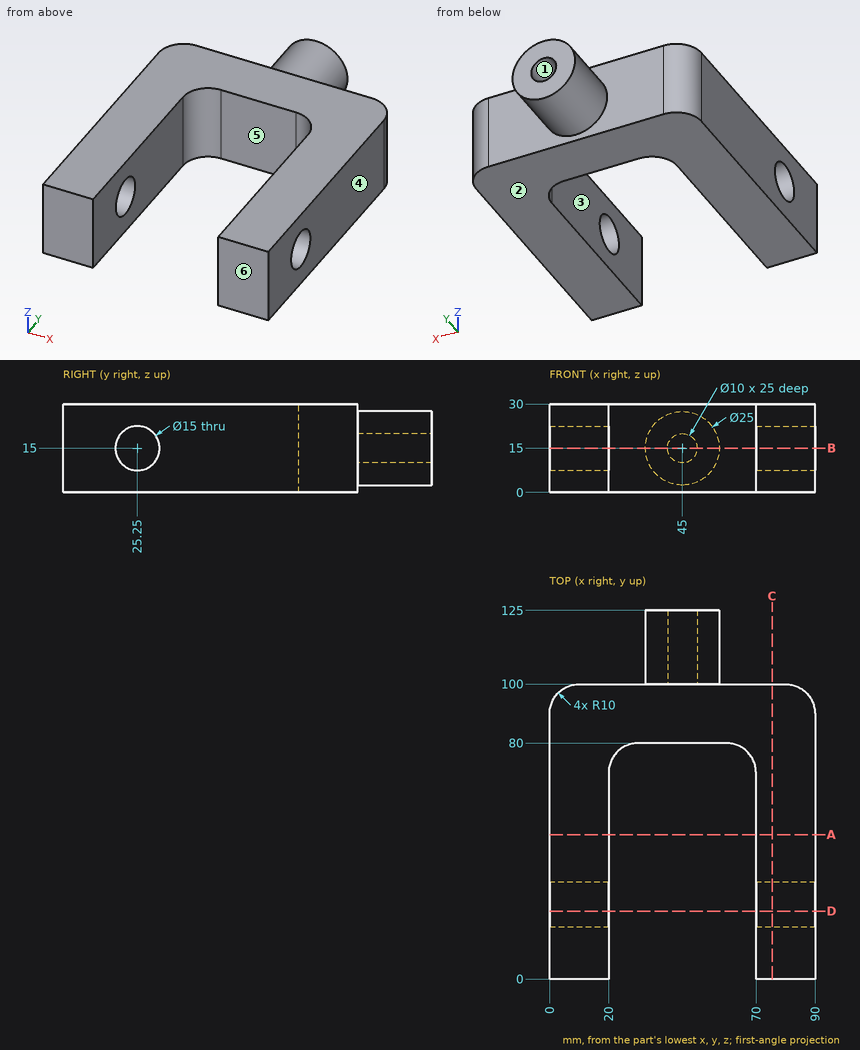
Source: three-view drawing plus pictorial views. Frame: mm from the lowest corner of the part. A direction names the side the tool comes from. Round coordinates to 2 decimals unless told otherwise and drop trailing zeros. Order: outer loops, then holes, each group sorted by start corner. A loop starts at its lowest first (then second) coordinate and runs counter-clockwise, first axis right, second up. Notation, with made-up numbers: (11, 16) - (15, 16) arc R18 ccw to (15, 26) - close; hole circle Ø4 at (-7.5, 58). An arc over 180 degrees is marked (long way). Write each question's results on one line, items separated by ' | '.
Item 1: Material intervals for line 1 along X through (y, z) = (11.5, 15.5); line 2 along X through (y, z) = (116, 15); line 3 along Y through (x, z) = (79.5, 27.75), sorted ascending. Write a range as [from, to].
Completed:
line 1: [0, 20], [70, 90] | line 2: [32.5, 40], [50, 57.5] | line 3: [0, 100]
Item 2: Section D-D, the plane y = 23. Return the cut outline in (x, z), and give its area (3 significant figures).
Completed:
outline: (0, 0) - (20, 0) - (20, 7.85) - (0, 7.85) - close; (0, 22.15) - (20, 22.15) - (20, 30) - (0, 30) - close; (70, 0) - (90, 0) - (90, 7.85) - (70, 7.85) - close; (70, 22.15) - (90, 22.15) - (90, 30) - (70, 30) - close | area: 628 mm^2
Item 3: Section A-A, the plane y = 49. Return the cut outline in (x, z), and give its area (3 significant figures).
Completed:
outline: (0, 0) - (20, 0) - (20, 30) - (0, 30) - close; (70, 0) - (90, 0) - (90, 30) - (70, 30) - close | area: 1,200 mm^2
Item 4: Section B-B, the plane z = 15. Return the cut outline in (x, y).
Completed:
outline: (0, 0) - (20, 0) - (20, 17.75) - (0, 17.75) - close; (0, 32.75) - (20, 32.75) - (20, 70) arc R10 cw to (30, 80) - (60, 80) arc R10 cw to (70, 70) - (70, 32.75) - (90, 32.75) - (90, 90) arc R10 ccw to (80, 100) - (57.5, 100) - (57.5, 125) - (50, 125) - (50, 100) - (40, 100) - (40, 125) - (32.5, 125) - (32.5, 100) - (10, 100) arc R10 ccw to (0, 90) - close; (70, 0) - (90, 0) - (90, 17.75) - (70, 17.75) - close
Item 5: Section C-C, the plane x = 75.5. Return the cut outline in (y, z), and give its area (3 significant figures).
Completed:
outline: (0, 0) - (100, 0) - (100, 30) - (0, 30) - close; hole circle Ø15 at (25.25, 15) | area: 2,820 mm^2
Item 6: Mould query, pull axis X, two halves, no side actions, for the marked faces 4, 5 and 6. Classes: pulls with the +X half, pulls with the -X half, needs draft (parallel to the pull), parting line crosses it, or undercut.
Completed:
face 4: pulls with the +X half | face 5: undercut | face 6: needs draft
Item 7: Reachability of the marked faces 1, 2 and 3 from +Z, -Z, +X, -X, +Y, -Y: full face, straight path, thin tool, end or side. Return the list, or none.
Completed:
face 1: +Y | face 2: -Z, +X, -X, +Y, -Y | face 3: +Z, -Z, -Y
Item 8: First-contact query: pin 1 Ø3 at (y, z) = (92, 11.5) entering from +X; pin 2 Ø16 at (x, z) = (45, 15) entering from -Y. Flat tips, straight axial feed; report the tip coordinate or a pass-through.
Completed:
pin 1: x = 89.99 | pin 2: y = 80
